Could you check a few things on this model? Use its own coordinates, in mm. A direction names the side the tool comes from. Give positions to 0.01 mm unless a question says otherwise; leave off trailing zeros. Loops run counter-clockwise (first coordinate to the right, second up) from the corner with the lowest first, then second, coordinate; pieces in that order, holes last.
1. I need wall thicknesses on line 1 along Z through (x, y) = (4, 12.5); line 2 along X through (y, z) = (-4, 7); line 3 along Y through (x, z) = (1, -14). Which ranges of each line are inside material? Lowest first, please.
2. Imagine slicing it at B-B (z = -49). List the corners of the cut face in (x, y) for me.
3. Imagine slicing it at D-D (x = 12). List the corners of the cut face in (y, z) for me, plus the area to 3 significant figures.
4. For P1, Ø12, axis at x = 10, z = -8, coming from the -Y side; P2, Ø5, axis at y = 2, z = -0.5, coming from the +X side; P3, Ø5, axis at x = -13, y = 0, coming from the -Z side; P4, Ø12, axis at y = 5.5, z = -26.5, coming from the +X side, each with a flat end and sliding along its axis, tell me the tip position at first contact or that it passes through.
5. For faces 1 (the cylindrical face through (-2.17, 9.76, -51.56)), 2 (the flat face through (0, 15, 7)), which set-ups out of +Z, -Z, +X, -X, +Y, -Y let a thin tool reach every point of the face, with its end or its side?
Solid Edge part; units mm, degrees
sketch "Sketch1" plane through (0, 0, 0) normal (0, 0, 1) x (1, 0, 0)
  circle A0 centre (0, 0) radius 17.4
extrude "Protrusion1" add sketch "Sketch1" along normal blind 12.88
sketch "Sketch2" plane through (0, 0, 0) normal (0, 0, -1) x (1, 0, 0)
  circle A0 centre (0, 0) radius 10
extrude "Protrusion2" add sketch "Sketch2" along normal blind 75
sketch "Sketch3" plane through (0, 0, -75) normal (0, 0, -1) x (1, 0, 0)
  circle A0 centre (0, 0) radius 9.9997
extrude "Cutout1" cut sketch "Sketch3" against normal blind 46 flip side to cut
chamfer "Chamfer_1" distance 1.5 angle 45 1 edges at (-9.9997, 0, -75)
sketch "Sketch4" plane through (0, 0, 12.88) normal (0, 0, 1) x (1, 0, 0)
  line L0 (-8.8182, 15) -> (8.8182, 15)
extrude "Cutout2" cut sketch "Sketch4" against normal up to next material side at (0, 15.05, 12.88)
pattern_circular "Pattern1" count 6 over 360 about axis through (0, 0, 12.88) along (0, 0, 1) of "Cutout2"
properties part number "185588"
Derived:
1. line 1: z = 0 to 12.88
1. line 2: x = -15.01 to 15.01
1. line 3: y = -9.95 to 9.95
2. outline: circle Ø20 at (0, 0)
3. outline: (-9.22, 0) - (9.22, 0) - (9.22, 12.88) - (-9.22, 12.88) - close
3. area: 237 mm2
4. P1: stops at y = -9.17
4. P2: stops at x = 17.32
4. P3: stops at z = 0
4. P4: stops at x = 10
5. face 1: -Z
5. face 2: +Z, -Z, +X, -X, +Y
